Here's how the part is built. I have some questions about the finished solid (model axes, mm). A direction names the side the tool comes from. Coordinates: 2 decimals unless noted, no trailing zeros. Write each loop counter-clockwise with the first axis right and the second up, starting at its lowest first coordinate (ties: lowest second). Pieces come first, ordered by that corner, then holes.
(1) Imagine slicing it at D-D, the plane z = 8. List the corners of the cut face in (x, y) for me, plus the area to 3 significant figures.
(2) Which directions (+Z, -Z, +X, -X, +Y, -Y) give clear straight access to the entire face, cutting with the end or side of a thin tool? Please do faces 1 (the flat face through (7, 3, 5)), 2 (the cylindrical face through (1.22, 8.68, 3.65)).
(3) For pin 1 Ø4 at (x, y) = (4, 6.5) entering from +Z; pin 2 Ø5 at (y, z) = (5.5, 4.5) entering from +X, each with a flat end and sliding along its axis, tell me the tip position at first contact or that it passes through.
(4) Please list where these lines run through material, in increasing order: probe 1 along Z at (x, y) = (0, -2); probe 2 along X at (y, z) = (4, 2.5); probe 3 along Z at (x, y) = (0, 7.5).
(5) Imagine slicing it at A-A, the plane x = 0. List the corners of the cut face in (y, z) for me.
(6) Thinking about a two-plate mould opening in Y: for faces 3 (the cylindrical face through (-3.88, 8.12, 2.54)), 4 (the cylindrical face through (8.77, -2.03, 2.54)), 5 (the flat face through (0, 0, 9)), 6 (the cylindrical face through (3.88, -8.12, 2.54)), which applies, released by +Y, released by -Y, zero draft, split by the parting line, or undercut?
```python
from build123d import *

# Parameters (mm, degrees)
SKETCH_R           = 8.5
PAD_DEPTH          = 5
PAD001_DEPTH       = 5
POLARPATTERN_COUNT = 14
SKETCH006_R        = 1.5
POCKET_DEPTH       = 9.001
POCKET_DEPTH_BACK  = -9.001


with BuildPart() as part:
    # Sketch → Pad (new body)
    with BuildSketch(Plane.XY):
        Circle(SKETCH_R)
    extrude(amount=PAD_DEPTH)

    # Sketch001 (on Face3 of Pad) → Pad001 (join)
    with BuildSketch(Plane.XY.offset(5)):
        with BuildLine():
            ThreePointArc((1.706561, 8.326923), (0, 9), (-1.706561, 8.326923))
            ThreePointArc((1.706561, 8.326923), (0, 8.5), (-1.706561, 8.326923))
        make_face()
    pad001 = extrude(amount=-PAD001_DEPTH)

    # PolarPattern: Pad001 ×14 about axis
    polarpattern_axis = Axis((0, 0, 5), (0, 0, 1))
    for i in range(1, POLARPATTERN_COUNT):
        add(pad001.rotate(polarpattern_axis, i * 360 / POLARPATTERN_COUNT))

    # Sketch006 → Pocket (cut, two sides)
    with BuildSketch(Plane.XZ) as pocket_sk:
        with Locations((0, 2.5)):
            Circle(SKETCH006_R)
    extrude(amount=-POCKET_DEPTH, mode=Mode.SUBTRACT)
    extrude(pocket_sk.sketch, amount=-POCKET_DEPTH_BACK, mode=Mode.SUBTRACT)

    # Sketch004 → Revolution (revolve)
    with BuildSketch(Plane.XZ):
        with BuildLine():
            Line((0, 5), (7.25, 5))
            ThreePointArc((6.25, 7), (6.131966, 5.690983), (7.25, 5))
            Line((6.25, 7), (5.25, 7))
            ThreePointArc((3, 9), (3.675934, 7.494801), (5.25, 7))
            Line((0, 9), (3, 9))
            Line((0, 9), (0, 7))
            Line((0, 7), (0, 5))
        make_face()
    revolve(axis=Axis((0, 0, 0), (0, 0, 1)))


solid = part.part
```
Recorded:
1. outline: circle Ø6.53 at (0, 0)
1. area: 33.5 mm2
2. face 1: +Z
2. face 2: +Z, -Z, +Y
3. pin 1: stops at z = 7
3. pin 2: stops at x = 8.3
4. probe 1: z = 0 to 1, 4 to 9
4. probe 2: x = -7.58 to -1.5, 1.5 to 7.58
4. probe 3: z = 0 to 1, 4 to 5
5. outline: (-9, 0) - (9, 0) - (9, 1) - (-9, 1) - close; (-9, 4) - (9, 4) - (9, 5) - (7.25, 5) arc R1.25 cw to (6.25, 7) - (5.25, 7) arc R2.01 cw to (3, 9) - (-3, 9) arc R2.01 cw to (-5.25, 7) - (-6.25, 7) arc R1.25 cw to (-7.25, 5) - (-9, 5) - close
6. face 3: released by +Y
6. face 4: undercut
6. face 5: zero draft
6. face 6: released by -Y
